Geometry check sheet. Reference: the model listing, model coordinates, mm. A direction names the side the tool comes from. Give positions to 0.01 mm unless a question says otherwise; leave off trailing zeros. Write each loop counter-clockwise with the first axis right and the second up, starting at its lowest first coordinate (ties: lowest second). Pieces come first, ordered by that corner, then holes. Notation, with made-up numbers: (80, 47.5) -> (133, 47.5) arc R20 ccw to (133, 76.5) -> close; hole circle Ø9 at (81, -37). An arc over 180 degrees is marked (long way). Use a Markdown table: item, result. Add a question column.
from build123d import *

# Parameters (mm, degrees)
ESBO_O1_R                = 5
RESSALTO_EXTRUS_O1_DEPTH = 6


with BuildPart() as part:
    # Esboço1 → Ressalto-extrusão1 (new body)
    with BuildSketch(Plane.XY):
        with BuildLine():
            Line((-72.5, 60), (-99.730887893, 60))
            ThreePointArc((-99.730887893, 60), (-103.240969816, 62.08184336), (-103.097331367, 66.160337553))
            ThreePointArc((-103.097331367, 66.160337553), (0, 122.5), (103.097331367, 66.160337553))
            ThreePointArc((103.097331367, 66.160337553), (103.240969816, 62.08184336), (99.730887893, 60))
            Line((99.730887893, 60), (72.5, 60))
            Line((72.5, 60), (72.5, -60))
            Line((72.5, -60), (99.730887893, -60))
            ThreePointArc((99.730887893, -60), (103.240969816, -62.08184336), (103.097331367, -66.160337553))
            ThreePointArc((103.097331367, -66.160337553), (0, -122.5), (-103.097331367, -66.160337553))
            ThreePointArc((-103.097331367, -66.160337553), (-103.240969816, -62.08184336), (-99.730887893, -60))
            Line((-99.730887893, -60), (-72.5, -60))
            Line((-72.5, -60), (-72.5, 60))
        make_face()
        with Locations((0, -30)):
            Circle(ESBO_O1_R, mode=Mode.SUBTRACT)
        Circle(ESBO_O1_R, mode=Mode.SUBTRACT)
        with Locations((0, 30)):
            Circle(ESBO_O1_R, mode=Mode.SUBTRACT)
    extrude(amount=RESSALTO_EXTRUS_O1_DEPTH)


solid = part.part
1) Tool access check on faces 1 (the face through (86, 60, 3)), 2 (the face through (-1.08, -4.88, 2.96)), 3 (the face through (-86, -60, 3)). Record the directions out of +Z, -Z, +X, -X, +Y, -Y that give a thin tool (end or side, any length) a straight path to the whole face; none if there is none.
2) Sectioned sample at A-A, the plane y = 0. Enter the section's corners in (x, z).
3) Sectioned sample at C-C, the plane z = 3.3. Enter the section's corners in (x, y).
4) Sectioned sample at B-B, the plane x = 0. Enter the section's corners in (y, z).
5) Draft check along X on faces 4 (the face through (103.21, -62.03, 2.96)), 5 (the face through (-86, 60, 3)), 6 (the face through (-1.08, -34.88, 2.96)). Enter one of: +X half, -X half, draft (parallel to the pull), parting line (faces both ways), or undercut.
6) Sectioned sample at D-D, the plane x = -89. Enter the section's corners in (y, z), and give its area (3 significant figures).
7) Material ranges on probe 1 along Y at (x, z) = (0, 2.85); probe 2 along X at (y, z) = (0.5, 0.3); probe 3 along X at (y, z) = (15.5, 5.75), recorded low to high. Write a range as [from, to].
8) Gauge pin test, flat ends, axial feed: P1, Ø1, axis at y = 22, z = 2, coming from the +X side; P2, Ø3, axis at x = -82.5, z = 3.5, coming from the +Y side; P3, Ø1.8, axis at y = 9.5, z = 2.5, coming from the -X side; P4, Ø6, axis at x = 28.5, y = -62, coming from the -Z side. Record the tip position at first contact, or that the pin passes through.
Check values:
| question | item | result |
|---|---|---|
| 1 | face 1 | +Z, -Z, +X |
| 1 | face 2 | +Z, -Z |
| 1 | face 3 | +Z, -Z, -X |
| 2 | outline | (-72.5, 0) -> (-5, 0) -> (-5, 6) -> (-72.5, 6) -> close; (5, 0) -> (72.5, 0) -> (72.5, 6) -> (5, 6) -> close |
| 3 | outline | (-103.1, -66.16) arc R122.5 ccw to (103.1, -66.16) arc R4 ccw to (99.73, -60) -> (72.5, -60) -> (72.5, 60) -> (99.73, 60) arc R4 ccw to (103.1, 66.16) arc R122.5 ccw to (-103.1, 66.16) arc R4 ccw to (-99.73, 60) -> (-72.5, 60) -> (-72.5, -60) -> (-99.73, -60) arc R4 ccw to start; hole circle Ø10 at (0, -30); hole circle Ø10 at (0, 0); hole circle Ø10 at (0, 30) |
| 4 | outline | (-122.5, 0) -> (-35, 0) -> (-35, 6) -> (-122.5, 6) -> close; (-25, 0) -> (-5, 0) -> (-5, 6) -> (-25, 6) -> close; (5, 0) -> (25, 0) -> (25, 6) -> (5, 6) -> close; (35, 0) -> (122.5, 0) -> (122.5, 6) -> (35, 6) -> close |
| 5 | face 4 | +X half |
| 5 | face 5 | draft |
| 5 | face 6 | undercut |
| 6 | outline | (-84.17, 0) -> (-60, 0) -> (-60, 6) -> (-84.17, 6) -> close; (60, 0) -> (84.17, 0) -> (84.17, 6) -> (60, 6) -> close |
| 6 | area | 290 mm² |
| 7 | probe 1 | [-122.5, -35], [-25, -5], [5, 25], [35, 122.5] |
| 7 | probe 2 | [-72.5, -4.97], [4.97, 72.5] |
| 7 | probe 3 | [-72.5, 72.5] |
| 8 | P1 | x = 72.5 |
| 8 | P2 | y = 91.9 |
| 8 | P3 | x = -72.5 |
| 8 | P4 | z = 0 |
